Geometry: see drawing. Coordinates: mm, zero at the bounding-box minimum. Round coordinates to 2 decimals unless told otherwise and drop trailing zeros. Loops run counter-clockwise (first coordinate to the right, second up) from the corner with the lowest first, then second, coordinate; pieces in that order, holes last. Notation, with made-up numbers: (46.25, 3.5) - (82.25, 3.5) arc R15 cw to (82.25, 22.5) - close; hole circle Ø8 at (86, 89.25). An arc over 180 degrees is marked (long way). Write item = value, one per line. Start each with the question number.
Item 1: Section A-A (z = 7). Return loops of the section in (x, y).
Item 2: Line query: line 1 (Z direction, x = 0.65, y = 11.8); line 2 (Y direction, x = 0.25, z = 40) (1 decimal); line 3 (Z direction, x = 1.3, y = 13.5) (1 decimal). Output: solid intervals per line, ascending. Write a range as from..to.
Item 3: First-contact query: pin 1 (1.5 mm diameter, centred on x = 1.5, z = 48, fed in from -Y); pin 2 (1 mm diameter, centred on x = 2, y = 10, fed in from +Z); pin 3 (1.5 mm diameter, centred on y = 5.6, z = 39.62, fed in from +X). Flat tips, straight axial feed; report the tip coordinate or a pass-through.
Item 4: Section D-D (y = 18). Return loops of the section in (x, z), plus the area to 3 significant figures.
Item 5: Section B-B (y = 12.5). Count the separate pieces of the cut face and the enclosed holes in it, plus the area to 3 significant figures.
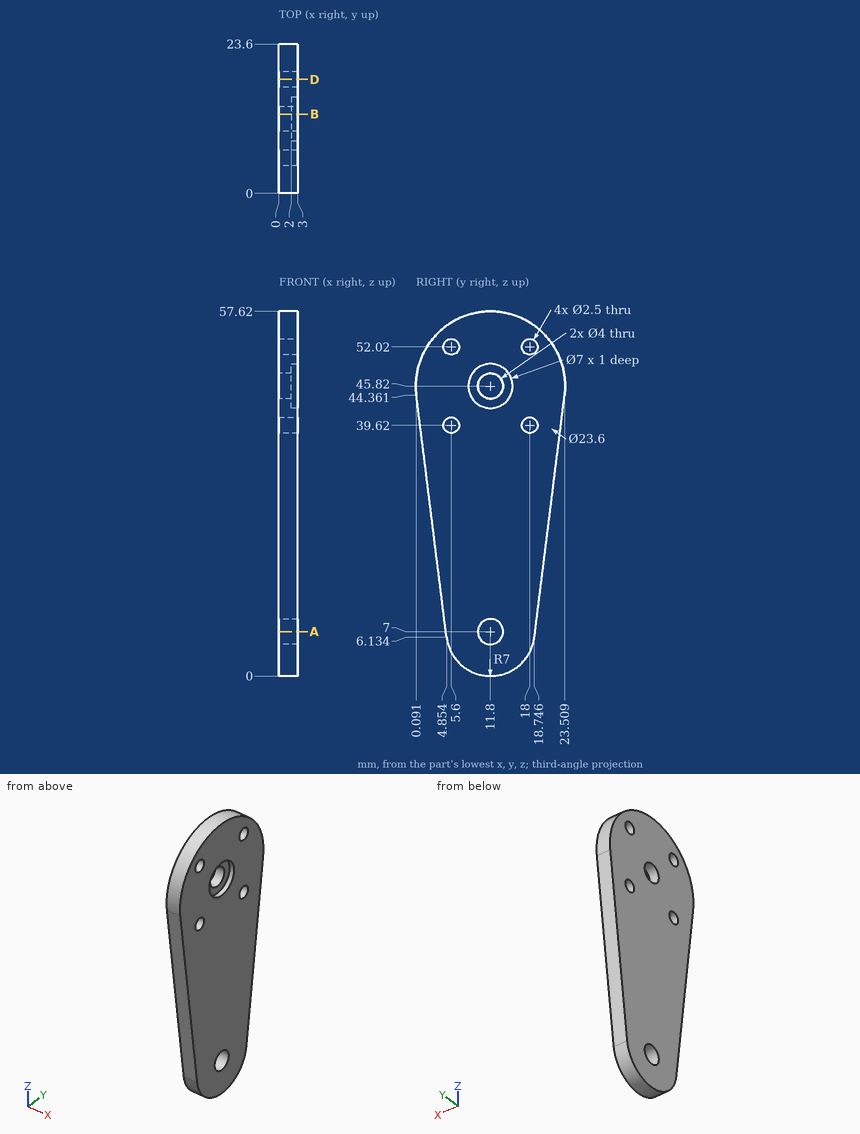
Taken from the geometry:
q1.outline = (0, 4.75) - (3, 4.75) - (3, 9.8) - (0, 9.8) - close; (0, 13.8) - (3, 13.8) - (3, 18.85) - (0, 18.85) - close
q2.line_1 = 0..5, 9..43.82, 47.82..57.62
q2.line_2 = 0.6..4.4, 6.8..16.8, 19.2..23
q2.line_3 = 0.2..5.9, 8.1..44.8, 46.9..57.5
q3.pin_1 = 0.09
q3.pin_2 = 57.55
q3.pin_3 = through
q4.outline = (0, 3.75) - (3, 3.75) - (3, 38.37) - (0, 38.37) - close; (0, 40.87) - (3, 40.87) - (3, 50.77) - (0, 50.77) - close; (0, 53.27) - (3, 53.27) - (3, 55.86) - (0, 55.86) - close
q4.area = 141 mm^2
q5.separate_pieces = 3
q5.enclosed_holes = 0
q5.area = 147 mm^2
